Geometry check sheet. Reference: the model listing, model coordinates, mm. A direction names the side the tool comes from. Coordinates: 2 decimals unless noted, no trailing zeros. Loops run counter-clockwise (first coordinate to the right, second up) from the corner with the lowest first, then second, coordinate; pieces in that order, holes last. Notation, with made-up numbers: (15.25, 67.25) -> (68.25, 67.25) arc R16 cw to (68.25, 80.25) -> close; hole circle Ø4 at (37, 16). An arc over 180 degrees is marked (long way). Answer as a JSON object with one key per item and string values.
Autodesk Inventor part; units mm, degrees
ref_plane "YZ Plane" through (0, 0, 0) normal (1, 0, 0) x (0, 1, 0)
ref_plane "XZ Plane" through (0, 0, 0) normal (0, 1, 0) x (-1, 0, 0)
ref_plane "XY Plane" through (0, 0, 0) normal (0, 0, 1) x (1, 0, 0)
sketch "Эскиз1" plane through (0, 0, 0) normal (0, 0, 1) x (1, 0, 0)
  line L0 (-18.25, -37.6) -> (18.25, -37.6)
  line L1 (18.25, -37.6) -> (18.25, 37.6)
  line L2 (18.25, 37.6) -> (-18.25, 37.6)
  line L3 (-18.25, 37.6) -> (-18.25, -37.6)
  line L4 (-18.25, 0) -> (18.25, 0) construction
  line L5 (0, 37.6) -> (0, -37.6) construction
  line L6 (-18.45, -37.8) -> (18.45, -37.8)
  line L7 (18.45, -37.8) -> (18.45, 37.8)
  line L8 (18.45, 37.8) -> (-18.45, 37.8)
  line L9 (-18.45, 37.8) -> (-18.45, -37.8)
  line L10 (-7.5, -37.8) -> (7.5, -37.8)
  line L11 (7.5, -37.8) -> (7.5, -40.8)
  line L12 (7.5, -40.8) -> (-7.5, -40.8)
  line L13 (-7.5, -40.8) -> (-7.5, -37.8)
  line L14 (-18.45, -37.8) -> (-18.45, -43.8)
  line L15 (-18.45, -43.8) -> (18.45, -43.8)
  line L16 (18.45, -43.8) -> (18.45, -37.8)
  line L17 (-18.45, 37.8) -> (-18.45, 43.8)
  line L18 (-18.45, 43.8) -> (18.45, 43.8)
  line L19 (18.45, 43.8) -> (18.45, 37.8)
  line L20 (-18.45, -43.8) -> (-21.45, -43.8)
  line L21 (-21.45, -43.8) -> (-21.45, 43.8)
  line L22 (-21.45, 43.8) -> (-18.45, 43.8)
  line L23 (-18.45, 43.8) -> (-18.45, -43.8)
  line L24 (18.45, 37.8) -> (18.45, 43.8)
  line L25 (21.45, -43.8) -> (21.45, 43.8)
  line L26 (21.45, 43.8) -> (18.45, 43.8)
  line L27 (18.45, 43.8) -> (18.45, -43.8)
  line L28 (7.5, 37.8) -> (7.5, 40.8)
  line L29 (7.5, 40.8) -> (-7.5, 40.8)
  line L30 (-7.5, 40.8) -> (-7.5, 37.8)
  line L31 (-21.45, -43.8) -> (-11.45, -43.8)
  line L32 (18.45, -43.8) -> (21.45, -43.8)
  line L33 (21.45, -43.8) -> (11.45, -43.8)
  line L34 (16.45, 46.7) -> (21.45, 46.7)
  line L35 (16.45, 46.7) -> (11.45, 46.7)
  line L36 (11.45, 46.7) -> (11.45, 43.8)
  line L37 (21.45, 46.7) -> (21.45, 43.8)
  line L38 (11.45, 43.8) -> (16.45, 43.8)
  circle A0 centre (16.45, 43.8) radius 2.1
  line L39 (-16.45, 46.7) -> (-21.45, 46.7)
  line L40 (-16.45, 46.7) -> (-11.45, 46.7)
  line L41 (-11.45, 46.7) -> (-11.45, 43.8)
  line L42 (-21.45, 46.7) -> (-21.45, 43.8)
  circle A1 centre (-16.45, 43.8) radius 2.1
  line L43 (16.45, -46.7) -> (21.45, -46.7)
  line L44 (16.45, -46.7) -> (11.45, -46.7)
  line L45 (11.45, -46.7) -> (11.45, -43.8)
  line L46 (21.45, -46.7) -> (21.45, -43.8)
  circle A2 centre (16.45, -43.8) radius 2.1
  line L47 (-11.45, -46.7) -> (-11.45, -43.8)
  line L48 (-16.45, -46.7) -> (-11.45, -46.7)
  line L49 (-16.45, -46.7) -> (-21.45, -46.7)
  line L50 (-21.45, -46.7) -> (-21.45, -43.8)
  circle A3 centre (-16.45, -43.8) radius 2.1
  line L51 (-18.45, -37.8) -> (-18.95, -37.8)
  line L52 (-18.95, -37.8) -> (-18.95, -38.3)
  line L53 (-18.95, -38.3) -> (-18.45, -38.3)
  line L54 (-18.45, -38.3) -> (-18.45, -37.8)
  line L55 (-18.95, -38.3) -> (18.95, -38.3)
  line L56 (18.95, -38.3) -> (18.95, 38.3)
  line L57 (18.95, 38.3) -> (-18.95, 38.3)
  line L58 (-18.95, 38.3) -> (-18.95, -38.3)
  point P0 (0, 0)
  point P1 (0, 0)
  point P2 (-1.9914, -32.8601)
  point P3 (0, -37.8)
  dimension "d0" = 36.5
  dimension "d1" = 75.2
  dimension "d4" = 36.9
  dimension "d5" = 75.6
  dimension "d6" = 15
  dimension "d7" = 3
  dimension "d9" = 6
  dimension "d10" = 3
  dimension "d18" = 5
  dimension "d19" = 4.2
  dimension "d27" = 0.5
  dimension "d28" = 0.5
  dimension "d29" = 37.9
  dimension "d30" = 76.6
extrude "Выдавливание1" add sketch "Эскиз1" along normal blind 25 contours L55 L13 L12 L11 L16 A2 L15 A3 L14 | L14 A3 L20 L21 L22 A1 L17 L57 L58 L52 L53 | L55 L11 L12 L13 | L17 A1 L18 A0 L19 L57 L28 L29 L30 | A3 L15 L14 | L14 L20 A3 | L30 L29 L28 L57 | A1 L22 L17 | L17 L18 A1 | L15 A3 L20 | L15 L47 L48 L49 L50 L20 A3 | L55 L56 L57 L19 A0 L26 L25 L32 A2 L16 | L22 A1 L18 | L22 L42 L39 L40 L41 L18 A1 | A2 L32 L16 | L16 L15 A2 | L15 A2 L32 L46 L43 L44 L45 | A0 L18 L19 | L19 L26 A0 | L32 A2 L15 | L36 L35 L34 L37 L26 A0 L18 | L18 A0 L26
extrude "Выдавливание2" cut sketch "Эскиз1" along normal blind 8 contours A3 L15 L14 | L14 L20 A3 | A1 L22 L17 | L17 L18 A1 | L15 A3 L20 | L22 A1 L18 | A2 L32 L16 | L16 L15 A2 | A0 L18 L19 | L19 L26 A0 | L32 A2 L15 | L18 A0 L26
extrude "Выдавливание3" cut sketch "Эскиз1" along normal blind 22.5 contours L6 L11 L55 L13 | L55 L11 L12 L13 | L30 L57 L28 L8 | L30 L29 L28 L57
fillet "Сопряжение1" radius 2 4 edges at (21.45, -46.7, 12.5) (-21.45, -46.7, 12.5) (-21.45, 46.7, 12.5) (21.45, 46.7, 12.5)
properties part number "fast_akkum"
1. Section check B-B, the plane x = 3.5. Record the boundary of the cut face in (y, z).
Evaluation:
{"outline": "(-43.8, 0) -> (-40.8, 0) -> (-40.8, 22.5) -> (-38.3, 22.5) -> (-38.3, 25) -> (-43.8, 25) -> close; (38.3, 22.5) -> (40.8, 22.5) -> (40.8, 0) -> (43.8, 0) -> (43.8, 25) -> (38.3, 25) -> close"}
2. Section check D-D, the plane z = 16. Record the boundary of the cut face in (x, y), then the cut area to 3 significant figures.
Evaluation:
{"outline": "(-21.45, -44.7) arc R2 ccw to (-19.45, -46.7) -> (-11.45, -46.7) -> (-11.45, -43.8) -> (11.45, -43.8) -> (11.45, -46.7) -> (19.45, -46.7) arc R2 ccw to (21.45, -44.7) -> (21.45, 44.7) arc R2 ccw to (19.45, 46.7) -> (11.45, 46.7) -> (11.45, 43.8) -> (-11.45, 43.8) -> (-11.45, 46.7) -> (-19.45, 46.7) arc R2 ccw to (-21.45, 44.7) -> close; hole (-18.95, -38.3) -> (-7.5, -38.3) -> (-7.5, -40.8) -> (7.5, -40.8) -> (7.5, -38.3) -> (18.95, -38.3) -> (18.95, 38.3) -> (7.5, 38.3) -> (7.5, 40.8) -> (-7.5, 40.8) -> (-7.5, 38.3) -> (-18.95, 38.3) -> close", "area": "892 mm^2"}
3. Depth check by flat-ended pin: P1, Ø0.8, axis at x = 2.5, y = -39, coming from the -Z side; P2, Ø1.3, axis at x = 17, y = 43.5, coming from the -Z side; P3, Ø7.5, axis at x = 1, z = 17, coming from the -Y side. Enter the tip coordinate at first touch or a pass-through.
Evaluation:
{"P1": "stops at z = 22.5", "P2": "stops at z = 8", "P3": "stops at y = -43.8"}
4. Section check C-C, the plane y = -33.5. Record the boundary of the cut face in (x, z), then the cut area to 3 significant figures.
Evaluation:
{"outline": "(-21.45, 0) -> (-18.95, 0) -> (-18.95, 25) -> (-21.45, 25) -> close; (18.95, 0) -> (21.45, 0) -> (21.45, 25) -> (18.95, 25) -> close", "area": "125 mm^2"}
5. Mould release check, pull along X, two halves, no side actions. Record for faces 1 (the face through (-19.2, -3.2, 0)), 2 (the face through (16, -44, 8)), 3 (the face through (20.85, -46.13, 12.68)): released by +X, released by -X, zero draft, split by the parting line, or undercut.
Evaluation:
{"face 1": "zero draft", "face 2": "undercut", "face 3": "released by +X"}
6. Thickness scan on probe 1 along Y at (x, z) = (-16.45, 3.5); probe 2 along Y at (x, z) = (-18, 14.25); probe 3 along Y at (x, z) = (-10, 1). Record the ranges inside material, lowest first. Write a range as from..to.
Evaluation:
{"probe 1": "y = -46.7..-45.9, -41.7..-38.3, 38.3..41.7, 45.9..46.7", "probe 2": "y = -46.7..-38.3, 38.3..46.7", "probe 3": "y = -43.8..-38.3, 38.3..43.8"}
7. Tool access check on faces 4 (the face through (-18.95, 1, 12)), 5 (the face through (7.5, -40, 11)), 6 (the face through (11.45, -45, 12)). Record the directions out of +Z, -Z, +X, -X, +Y, -Y that give a thin tool (end or side, any length) a straight path to the whole face; none if there is none.
Evaluation:
{"face 4": "+Z, -Z", "face 5": "-Z", "face 6": "+Z, -Z, -Y"}
8. Section check A-A, the plane z = 6. State how many separate pieces and enclosed holes the cut face has, then the cut area to 3 significant figures.
Evaluation:
{"separate pieces": "1", "enclosed holes": "5", "area": "837 mm^2"}
